Work out the finished part from the listing and answer in its coordinate system (mm). A direction names the side the tool comes from. Coordinates: 2 decimals unless noted, no trailing zeros. Order: outer loops, then holes, each group sorted by start corner. A loop starts at its lowest first (then second) coordinate and runs counter-clockwise, first axis right, second up. Notation, with made-up numbers: M 87,-22 L 103,-22 A17 cw 103,-16 Z; hole C 7.5,61 d7. An arc over 180 degrees is marked long. Answer in a Markdown table with one row per item. Add a question column.
Item 1: The part is cut by section A-A (y = 30). Write down the section's boundary in (x, z).
Item 2: Flat-ended cylindrical pins translate along their axes: pin 1 Ø12 at (x, z) = (55, 34) entering from -Y (1 decimal); pin 2 Ø0.6 at (x, z) = (-47.5, 47.5) entering from -Y. Find the tip coordinate at first contact, or state that the pin passes through.
Item 3: The mould has two halves that part along Z. Classify faces 5 (the face through (1, 23, 50)), 6 (the face through (24, 22, 45)), 7 (the face through (-51.82, 14.76, 47.54)): released by +Z, released by -Z, zero draft, split by the parting line, or undercut.
Item 4: Which of the six approach directions +Z, -Z, +X, -X, +Y, -Y give full straight-line access (tool end or side, diameter ignored) to faces 1 (the face through (-1, 22, -50)), 2 (the face through (-72.54, 32.95, -28.12)), 3 (the face through (-51.892, 21.173, 47.535)), 4 (the face through (-20, 22, 1))?
Item 5: The part is cut by section C-C (x = 6). Write down the section's boundary in (y, z).
Item 6: Consider line 1 (X direction, y = 40, z = -12); line 2 (Y direction, x = -72.55, z = -30); line 3 (X direction, y = 29.5, z = -33). Determine where each line is inside the solid, lowest interval first. Write a range as from..to.
Item 7: The part is cut by section B-B (z = -43). Write down the section's boundary in (x, y), then the cut area to 3 significant figures.
Item 8: The part is cut by section D-D (z = -30). Write down the section's boundary in (x, y).
from build123d import *

# Parameters (mm, degrees)
SKETCH2_W           = 150
SKETCH2_H           = 100
SKETCH2_W_2         = 140
SKETCH2_H_2         = 90
BOSS_EXTRUDE3_DEPTH = 45
FILLET1_R           = 5
SKETCH3_W           = 5
SKETCH3_H           = 90
BOSS_EXTRUDE4_DEPTH = 45
SKETCH5_W           = 12
SKETCH5_H           = 9
CUT_EXTRUDE1_DEPTH  = 5
FILLET2_R           = 5
SKETCH6_R           = 3.5
CUT_EXTRUDE2_DEPTH  = 5


with BuildPart() as part:
    # Sketch2 → Boss-Extrude3 (new body)
    with BuildSketch(Plane(origin=(0, 0, 0), x_dir=(1, 0, 0), z_dir=(0, 1, 0))):
        Rectangle(SKETCH2_W, SKETCH2_H)
        Rectangle(SKETCH2_W_2, SKETCH2_H_2, mode=Mode.SUBTRACT)
    extrude(amount=BOSS_EXTRUDE3_DEPTH)

    # Fillet1
    fillet1_edges = [part.edges().sort_by_distance(p)[0] for p in [
        (75, 22.5, 50),
        (-75, 22.5, 50),
        (-75, 22.5, -50),
        (75, 22.5, -50),
    ]]
    fillet(fillet1_edges, radius=FILLET1_R)

    # Sketch3 → Boss-Extrude4 (add)
    with BuildSketch(Plane(origin=(0, 0, 0), x_dir=(1, 0, 0), z_dir=(0, 1, 0))):
        with Locations((-22.5, 0)):
            Rectangle(SKETCH3_W, SKETCH3_H)
    extrude(amount=BOSS_EXTRUDE4_DEPTH)

    # Sketch5 → Cut-Extrude1 (cut)
    with BuildSketch(Plane.XY.offset(50)):
        with Locations((-47.5, 18)):
            Rectangle(SKETCH5_W, SKETCH5_H)
    extrude(amount=-CUT_EXTRUDE1_DEPTH, mode=Mode.SUBTRACT)

    # Fillet2
    # the kernel refuses this fillet: 5 mm, written as the material it adds along each edge
    with BuildSketch(Plane(origin=(-53.5, 13.5, 50), x_dir=(0, 1, 0), z_dir=(0, 0, -1))) as fillet2_piece_1:
        with BuildLine():
            CenterArc((FILLET2_R, FILLET2_R), FILLET2_R, 180, 90)
            Line((0, FILLET2_R), (0, 0))
            Line((0, 0), (FILLET2_R, 0))
        make_face()
    extrude(amount=5)
    with BuildSketch(Plane(origin=(-53.5, 22.5, 50), x_dir=(0, -1, 0), z_dir=(0, 0, -1)), Plane(origin=(-41.5, 22.5, 50), x_dir=(-1, 0, 0), z_dir=(0, 0, -1)), Plane(origin=(-41.5, 13.5, 50), x_dir=(0, 1, 0), z_dir=(0, 0, -1))) as fillet2_piece_2:
        with BuildLine():
            CenterArc((FILLET2_R, -FILLET2_R), FILLET2_R, 90, 90)
            Line((0, -FILLET2_R), (0, 0))
            Line((0, 0), (FILLET2_R, 0))
        make_face()
    extrude(amount=5)

    # Sketch6 → Cut-Extrude2 (cut)
    with BuildSketch(Plane.ZY.offset(75)):
        with Locations((-30, 30)):
            Circle(SKETCH6_R)
    extrude(amount=-CUT_EXTRUDE2_DEPTH, mode=Mode.SUBTRACT)


solid = part.part
Reply:
| question | item | result |
|---|---|---|
| 1 | outline | M -75,-45 A5 ccw -70,-50 L 70,-50 A5 ccw 75,-45 L 75,45 A5 ccw 70,50 L -70,50 A5 ccw -75,45 L -75,-26.5 L -70,-26.5 L -70,45 L -25,45 L -25,-45 L -70,-45 L -70,-33.5 L -75,-33.5 Z; hole M -20,-45 L 70,-45 L 70,45 L -20,45 Z |
| 2 | pin 1 | passes through |
| 2 | pin 2 | stops at y = 0 |
| 3 | face 5 | released by +Z |
| 3 | face 6 | undercut |
| 3 | face 7 | zero draft |
| 4 | face 1 | -Z, +X, -X, +Y, -Y |
| 4 | face 2 | -X |
| 4 | face 3 | +Z |
| 4 | face 4 | +Y, -Y |
| 5 | outline | M 0,-50 L 45,-50 L 45,-45 L 0,-45 Z; M 0,45 L 45,45 L 45,50 L 0,50 Z |
| 6 | line 1 | x = -75..-70, -25..-20, 70..75 |
| 6 | line 2 | y = 0..26.5, 33.5..45 |
| 6 | line 3 | x = -25..-20, 70..75 |
| 7 | outline | M -75,0 L -70,0 L -70,45 L -75,45 Z; M -25,0 L -20,0 L -20,45 L -25,45 Z; M 70,0 L 75,0 L 75,45 L 70,45 Z |
| 7 | area | 675 mm2 |
| 8 | outline | M -75,0 L -70,0 L -70,26.5 L -75,26.5 Z; M -75,33.5 L -70,33.5 L -70,45 L -75,45 Z; M -25,0 L -20,0 L -20,45 L -25,45 Z; M 70,0 L 75,0 L 75,45 L 70,45 Z |
